Build history of the part. All positions in model axes, mm. Face numbers are marked on the shaded views. A direction names the side the tool comes from. Round coordinates to 2 decimals unless told otherwise and drop trailing zeros. Write item = value, one per line.
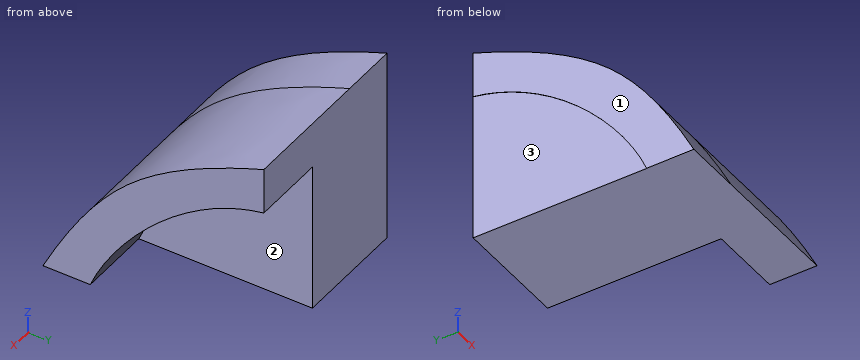
from build123d import *

# Parameters (mm, degrees)
F3_DEPTH      = 5.075
F4_DEPTH      = 11.7
F4_DEPTH_BACK = 5.1


# Not quite as in the source:
# - the program builds the solid bodies; features that only make, move or delete a surface that nothing else refers to are left out


with BuildPart() as f3:
    # F2 (on Right) → F3 (new body, symmetric)
    with BuildSketch(Plane.YZ):
        with BuildLine():
            Line((-28.3462911332, -4.9449687588), (-28.3462911332, 8.3612054586))
            add(Edge.make_bspline(
                [(-43.7509737622, -4.9449687588), (-41.7884092148, 0), (-35.7711096695, 7.1036480367), (-28.3462911332, 8.3612054586)],
                knots=[0, 0, 0, 0, 20.3557981716, 20.3557981716, 20.3557981716, 20.3557981716], degree=3))
            Line((-43.7509737622, -4.9449687588), (-28.3462911332, -4.9449687588))
        make_face()
    extrude(amount=F3_DEPTH, both=True)

    # F2 (on Right) → F4 (join, two sides)
    with BuildSketch(Plane.YZ) as f4_sk:
        with BuildLine():
            Line((-28.3462911332, 8.3612054586), (-28.3462911332, 12.4550312412))
            add(Edge.make_bspline(
                [(-47.9462911332, -4.9449687588), (-46.2080227994, -1.5012717921), (-41.5989810613, 6.6616658975), (-33.5069069781, 10.6230272322), (-28.3462911332, 12.4550312412)],
                knots=[0, 0, 0, 0, 0.4814819879, 1, 1, 1, 1], degree=3))
            Line((-47.9462911332, -4.9449687588), (-43.7509737622, -4.9449687588))
            add(Edge.make_bspline(
                [(-43.7509737622, -4.9449687588), (-41.7884092148, 0), (-35.7711096695, 7.1036480367), (-28.3462911332, 8.3612054586)],
                knots=[0, 0, 0, 0, 20.3557981716, 20.3557981716, 20.3557981716, 20.3557981716], degree=3))
        make_face()
    extrude(amount=F4_DEPTH)
    extrude(f4_sk.sketch, amount=-F4_DEPTH_BACK)


solid = f3.part
Q1. Which spindle directions (+Z, -Z, +X, -X, +Y, -Y) get a long thin tool onto all of the face, cutting with end or side? Do the marked faces 1, 2 and 3. Say none if no direction does.
Check values:
face_1 = +Z, -Z, -X, +Y, -Y
face_2 = -Z, +X, +Y
face_3 = -Z, -X, +Y
Q2. Flat gauge pins, fed straight in: pin 1 (5 mm diameter, centred on x = 3, z = -2.5, fed in from -Y); pin 2 (10 mm diameter, centred on x = 9, z = 3, fed in from -Y); pin 3 (6 mm diameter, centred on x = 6, y = -40.5, fed in from +Z); pin 4 (1 mm diameter, centred on y = -36.5, z = 10, fed in from +X). Where does each tip first touch, or does it go through?
Check values:
pin_1 = -47.95
pin_2 = -46.38
pin_3 = 8.15
pin_4 = through
Q3. Probe probe 1 along X at (y, z) = (-37.5, 2.5) (3 decimals); probe 2 along Z at (x, y) = (0.25, -37.75); probe 3 along Z at (x, y) = (5.5, -42.25). List the from-to ranges inside material, lowest first.
Check values:
probe_1 = -5.075 to 5.075
probe_2 = -4.94 to 7.99
probe_3 = -2.01 to 4.02
